Check sheet for the modelled part. Datum: model origin and axes. Units: mm. A direction names the side the tool comes from. Coordinates: 2 decimals unless noted, no trailing zeros. Loops run counter-clockwise (first coordinate to the right, second up) from the corner with the lowest first, then second, coordinate; pieces in that order, holes last.
```python
from build123d import *

# Parameters (mm, degrees)
SKETCH1_R           = 4
BOSS_EXTRUDE1_DEPTH = 14.25
SKETCH3_W           = 10
SKETCH3_H           = 20.5
CUT_EXTRUDE1_DEPTH  = 25
CUT_EXTRUDE2_DEPTH  = 19.3
CUT_EXTRUDE3_DEPTH  = 5.7
SKETCH7_R           = 3
CUT_EXTRUDE4_DEPTH  = 4.5000001


with BuildPart() as part:
    # Sketch1 → Boss-Extrude1 (new body, symmetric)
    with BuildSketch(Plane.XY):
        with BuildLine():
            Line((-35, 0), (35, 0))
            ThreePointArc((35, 0), (39.914888853, 8.179748676), (35, 16.359497352))
            Line((35, 16.359497352), (12.167035368, 28.5))
            Line((12.167035368, 28.5), (-42.832964632, 28.5))
            ThreePointArc((-42.832964632, 28.5), (-52.310648732, 21.689593093), (-48.878955781, 10.53470082))
            Line((-48.878955781, 10.53470082), (-35, 0))
        make_face()
        with Locations((12.167035368, 18.5)):
            Circle(SKETCH1_R, mode=Mode.SUBTRACT)
        with Locations((-33.832964632, 18.5)):
            Circle(SKETCH1_R, mode=Mode.SUBTRACT)
    extrude(amount=BOSS_EXTRUDE1_DEPTH, both=True)

    # Sketch3 → Cut-Extrude1 (cut)
    with BuildSketch(Plane(origin=(0, 28.5, 0), x_dir=(1, 0, 0), z_dir=(0, 1, 0))):
        with BuildLine():
            Line((-28.832964632, 10.25), (-42.832964632, 10.25))
            Line((-42.832964632, 10.25), (-42.832964632, -10.25))
            Line((-42.832964632, -10.25), (-28.832964632, -10.25))
            ThreePointArc((-28.832964632, -10.25), (-27.41875107, -9.664213562), (-26.832964632, -8.25))
            Line((-26.832964632, -8.25), (-26.832964632, 8.25))
            ThreePointArc((-26.832964632, 8.25), (-27.41875107, 9.664213562), (-28.832964632, 10.25))
        make_face()
        with Locations((-47.832964632, 0)):
            Rectangle(SKETCH3_W, SKETCH3_H)
    extrude(amount=-CUT_EXTRUDE1_DEPTH, mode=Mode.SUBTRACT)

    # Sketch3<3> → Cut-Extrude2 (cut)
    with BuildSketch(Plane(origin=(0, 28.5, 0), x_dir=(1, 0, 0), z_dir=(0, 1, 0))):
        with BuildLine():
            Line((-20.832964632, 10.25), (33.414888853, 10.25))
            ThreePointArc((33.414888853, 10.25), (34.829102415, 9.664213562), (35.414888853, 8.25))
            Line((35.414888853, 8.25), (35.414888853, -8.25))
            ThreePointArc((35.414888853, -8.25), (34.829102415, -9.664213562), (33.414888853, -10.25))
            Line((33.414888853, -10.25), (-20.832964632, -10.25))
            ThreePointArc((-20.832964632, -10.25), (-22.247178195, -9.664213562), (-22.832964632, -8.25))
            Line((-22.832964632, -8.25), (-22.832964632, 8.25))
            ThreePointArc((-22.832964632, 8.25), (-22.247178195, 9.664213562), (-20.832964632, 10.25))
        make_face()
    extrude(amount=-CUT_EXTRUDE2_DEPTH, mode=Mode.SUBTRACT)

    # Sketch6 → Cut-Extrude3 (cut)
    with BuildSketch(Plane(origin=(0, 9.2, 0), x_dir=(1, 0, 0), z_dir=(0, 1, 0))):
        with BuildLine():
            Line((-18.48327062, 3.406663741), (-14.359422457, 9.38555458))
            ThreePointArc((-14.359422457, 9.38555458), (-13.64281361, 10.020749723), (-12.71305804, 10.25))
            Line((-12.71305804, 10.25), (25.29498226, 10.25))
            ThreePointArc((25.29498226, 10.25), (26.22473783, 10.020749723), (26.941346678, 9.38555458))
            Line((26.941346678, 9.38555458), (31.06519484, 3.406663741))
            ThreePointArc((31.06519484, 3.406663741), (32.126101588, 0), (31.06519484, -3.406663741))
            Line((31.06519484, -3.406663741), (26.941346678, -9.38555458))
            ThreePointArc((26.941346678, -9.38555458), (26.22473783, -10.020749723), (25.29498226, -10.25))
            Line((25.29498226, -10.25), (-12.71305804, -10.25))
            ThreePointArc((-12.71305804, -10.25), (-13.64281361, -10.020749723), (-14.359422457, -9.38555458))
            Line((-14.359422457, -9.38555458), (-18.48327062, -3.406663741))
            ThreePointArc((-18.48327062, -3.406663741), (-19.544177367, 0), (-18.48327062, 3.406663741))
        make_face()
    extrude(amount=-CUT_EXTRUDE3_DEPTH, mode=Mode.SUBTRACT)

    # Sketch7 → Cut-Extrude4 (cut, through all)
    with BuildSketch(Plane(origin=(0, 3.5, 0), x_dir=(1, 0, 0), z_dir=(0, 1, 0))):
        with Locations((26.714888853, 0)):
            Circle(SKETCH7_R)
        with Locations((-13.285111147, 0)):
            Circle(SKETCH7_R)
    extrude(amount=-CUT_EXTRUDE4_DEPTH, mode=Mode.SUBTRACT)


solid = part.part
```
1) Section check A-A on z = -11.75. Enter the section's corners in (x, y), plus the area to 3 significant figures.
Answer sheet:
outline: (-48.88, 10.53) - (-35, 0) - (35, 0) arc R9.26 ccw to (35, 16.36) - (12.17, 28.5) - (-42.83, 28.5) arc R10 ccw to start; hole circle Ø8 at (-33.83, 18.5); hole circle Ø8 at (12.17, 18.5)
area: 2,180 mm2
2) Scan lines: line 1 (Z direction, x = 6, y = 17.75); line 2 (X direction, y = 18.5, z = 12.1); line 3 (X direction, y = 26.75, z = -1.75). Record each from-to range of solid material in increasing order.
Answer sheet:
line 1: z = -14.25 to -10.25, 10.25 to 14.25
line 2: x = -52.83 to -37.83, -29.83 to 8.17, 16.17 to 30.97
line 3: x = -26.83 to -22.83
3) Section check B-B on x = 10. Enter the section's corners in (y, z).
Answer sheet:
outline: (0, -14.25) - (15.14, -14.25) - (15.14, -10.25) - (3.5, -10.25) - (3.5, 10.25) - (15.14, 10.25) - (15.14, 14.25) - (0, 14.25) - close; (21.86, -14.25) - (28.5, -14.25) - (28.5, -10.25) - (21.86, -10.25) - close; (21.86, 10.25) - (28.5, 10.25) - (28.5, 14.25) - (21.86, 14.25) - close
4) Section check C-C on z = 0. Enter the section's corners in (x, y).
Answer sheet:
outline: (-39.61, 3.5) - (-35, 0) - (-16.29, 0) - (-16.29, 3.5) - (-19.54, 3.5) - (-19.54, 9.2) - (-22.83, 9.2) - (-22.83, 28.5) - (-26.83, 28.5) - (-26.83, 3.5) - close; (-10.29, 0) - (23.71, 0) - (23.71, 3.5) - (-10.29, 3.5) - close; (29.71, 0) - (35, 0) arc R9.26 ccw to (35.41, 16.13) - (35.41, 9.2) - (32.13, 9.2) - (32.13, 3.5) - (29.71, 3.5) - close
5) Set-up check for faces 1 (the cylindrical face through (-31.68, 21.87, -12.28)), 2 (the flat face through (35.415, 13, 0)), 3 (the flat face through (-41, 16, 10.25)): record each of +Z, -Z, +X, -X, +Y, -Y from which the full face is reachable in a straight line by a thin tool's end or side.
Answer sheet:
face 1: +Z, -Z
face 2: +Y
face 3: -X, +Y
6) Section check D-D on x = -41. Enter the section's corners in (y, z), plus the area to 3 significant figures.
Answer sheet:
outline: (4.55, -14.25) - (28.5, -14.25) - (28.5, -10.25) - (4.55, -10.25) - close; (4.55, 10.25) - (28.5, 10.25) - (28.5, 14.25) - (4.55, 14.25) - close
area: 192 mm2
7) Depth check by flat-ended pin: pin 1 (1.5 mm diameter, centred on x = 10, z = -6.5, fed in from +Y); pin 2 (1.5 mm diameter, centred on y = 22, z = 9, fed in from +X); pin 3 (5.5 mm diameter, centred on x = -13.29, z = 0, fed in from +Y); pin 4 (5 mm diameter, centred on y = 19, z = 1, fed in from -X). Enter the tip coordinate at first touch or a pass-through.
Answer sheet:
pin 1: stops at y = 3.5
pin 2: stops at x = -22.16
pin 3: passes through
pin 4: stops at x = -26.83
8) Mould release check, pull along Y, two halves, no side actions. Record for faces 4 (the cylindrical face through (-31.68, 21.87, 12.22)), 5 (the cylindrical face through (11.646, 22.466, 12.222)), 6 (the cylindrical face through (23.718, 1.774, -0.132)), 7 (the cylindrical face through (-52.254, 21.854, -12.222)): +Y half, -Y half, draft (parallel to the pull), parting line (faces both ways), or undercut.
Answer sheet:
face 4: undercut
face 5: undercut
face 6: draft
face 7: parting line
